Design review of the part built by this model. Coordinates are the model's own, in mm. A direction names the side the tool comes from. Coordinates: 2 decimals unless noted, no trailing zeros. Order: outer loops, then holes, each group sorted by start corner. A loop starts at its lowest first (then second) coordinate and runs counter-clockwise, first axis right, second up.
from build123d import *

# Parameters (mm, degrees)
SKETCH_1_W          = 42
SKETCH_1_H          = 42
EXTRUDE_1_DEPTH     = 40
CHAMFER_1_SIZE      = 5
SKETCH_2_R          = 11
EXTRUDE_2_DEPTH     = 2
SKETCH_3_R          = 2.5
EXTRUDE_3_DEPTH     = 23
SKETCH_4_R          = 1.75
CUT_EXTRUDE_1_DEPTH = 3


with BuildPart() as part:
    # 草圖1 → 填料-伸長1 (new body)
    with BuildSketch(Plane.XY):
        Rectangle(SKETCH_1_W, SKETCH_1_H)
    extrude(amount=EXTRUDE_1_DEPTH)

    # 導角1
    chamfer_1_edges = [part.edges().sort_by_distance(p)[0] for p in [
        (-21, 21, 20),
        (21, 21, 20),
        (21, -21, 20),
        (-21, -21, 20),
    ]]
    chamfer(chamfer_1_edges, length=CHAMFER_1_SIZE)

    # 草圖2 → 填料-伸長2 (add)
    with BuildSketch(Plane.XY.offset(40)):
        Circle(SKETCH_2_R)
    extrude(amount=EXTRUDE_2_DEPTH)

    # 草圖3 → 填料-伸長3 (add)
    with BuildSketch(Plane.XY.offset(42)):
        Circle(SKETCH_3_R)
    extrude(amount=EXTRUDE_3_DEPTH)

    # 草圖4 → 除料-伸長1 (cut)
    with BuildSketch(Plane.XY.offset(40)):
        with Locations((-15.5, 15.5)):
            Circle(SKETCH_4_R)
        with Locations(Location((-15.5, -15.5, 0), (0, 0, 180))):
            Circle(SKETCH_4_R)
        with Locations((15.5, -15.5)):
            Circle(SKETCH_4_R)
        with Locations(Location((15.5, 15.5, 0), (0, 0, 180))):
            Circle(SKETCH_4_R)
    extrude(amount=-CUT_EXTRUDE_1_DEPTH, mode=Mode.SUBTRACT)


solid = part.part
1. Add section A-A (z = 24). Give the boundary of the cut face in (x, y).
2. Mouldability with a two-part tool opening along X and no side actions: class faces 3 (the cylindrical face through (14.6, 14, 38.5)), 4 (the flat face through (18, 19, 20)), 5 (the flat face through (0, 0, 0)) as pulls with the +X half, pulls with the -X half, needs draft (parallel to the pull), parting line crosses it, or undercut.
3. For faces 1 (the flat face through (-15, -16, 37)), 2 (the flat face through (-18, 19, 20)), list the 3-axis set-ups (+Z, -Z, +X, -X, +Y, -Y) from which the entire face can be reached by the end or side of a thin tool; tool diameter is ignored.
4. Add section B-B (x = 0). Give the boundary of the cut face in (y, z), and give its area (3 significant figures).
5. Add section D-D (y = -8.5). Give the boundary of the cut face in (x, z), and give its area (3 significant figures).
6. Insertion check: pin 1 (1 mm diameter, centred on x = -15, y = -15, fed in from +Z); pin 2 (6 mm diameter, centred on x = 10.5, y = 3, fed in from +Z); pin 3 (10 mm diameter, centred on x = 11.5, y = 13, fed in from -Z); pin 4 (4 mm diameter, centred on x = -15.5, y = -15.5, fed in from +Z). Each pin has a flat end and moves straight along its axis. Give the tip position at first contact, or say it passes through.
7. To check wall thickness, follow line 1 (Y direction, x = 15.5, z = 38.1); line 2 (Z direction, x = -5, y = 18); line 3 (Z direction, x = 9, y = -5.5). State the ranges of each line that lie inside material, in increasing order.
Solution:
1. outline: (-21, -16) - (-16, -21) - (16, -21) - (21, -16) - (21, 16) - (16, 21) - (-16, 21) - (-21, 16) - close
2. face 3: undercut
2. face 4: pulls with the +X half
2. face 5: needs draft
3. face 1: +Z
3. face 2: +Z, -Z, -X, +Y
4. outline: (-21, 0) - (21, 0) - (21, 40) - (11, 40) - (11, 42) - (2.5, 42) - (2.5, 65) - (-2.5, 65) - (-2.5, 42) - (-11, 42) - (-11, 40) - (-21, 40) - close
4. area: 1,840 mm2
5. outline: (-21, 0) - (21, 0) - (21, 40) - (6.98, 40) - (6.98, 42) - (-6.98, 42) - (-6.98, 40) - (-21, 40) - close
5. area: 1,710 mm2
6. pin 1: stops at z = 37
6. pin 2: stops at z = 42
6. pin 3: stops at z = 0
6. pin 4: stops at z = 40
7. line 1: y = -21 to -17.25, -13.75 to 13.75, 17.25 to 21
7. line 2: z = 0 to 40
7. line 3: z = 0 to 42
